Design review of the part built by this model. Coordinates are the model's own, in mm. A direction names the side the tool comes from. Give positions to 0.01 mm unless a question says otherwise; leave off trailing zeros. Order: outer loops, then holes, each group sorted by start corner. A loop starts at its lowest first (then second) coordinate and runs counter-clockwise, first axis right, second up.
```python
from build123d import *

# Parameters (mm, degrees)
BASE_FLANGE1_DEPTH = 40
SKETCH2_R          = 13
CUT_EXTRUDE1_DEPTH = 115.512008104
SKETCH3_R          = 13
CUT_EXTRUDE2_DEPTH = 117.704755687
SKETCH4_R          = 3
CUT_EXTRUDE3_DEPTH = 10
SKETCH5_R          = 3
CUT_EXTRUDE4_DEPTH = 10


# Sheet-metal steps are written as plain solids
with BuildPart() as part:
    # Sketch1 → Base-Flange1 (new body)
    with BuildSketch(Plane.XY):
        with BuildLine():
            Line((0, 0), (-80, 0))
            ThreePointArc((-80, 0), (-82.121320344, -0.878679656), (-83, -3))
            Line((-83, -3), (-83, -68))
            Line((-83, -68), (-86, -68))
            Line((-86, -68), (-86, -3))
            ThreePointArc((-86, -3), (-84.242640687, 1.242640687), (-80, 3))
            Line((-80, 3), (0, 3))
            Line((0, 3), (0, 0))
        make_face()
    extrude(amount=BASE_FLANGE1_DEPTH)

    # Sketch2 → Cut-Extrude1 (cut, through all)
    with BuildSketch(Plane(origin=(-83, 0, 0), x_dir=(0, 0, -1), z_dir=(1, 0, 0))):
        with Locations(Location((-20, -25, 0), (0, 0, 90))):
            Circle(SKETCH2_R)
    extrude(amount=-CUT_EXTRUDE1_DEPTH, mode=Mode.SUBTRACT)

    # Sketch3 → Cut-Extrude2 (cut, through all)
    with BuildSketch(Plane.XZ):
        with Locations((-36, 20)):
            Circle(SKETCH3_R)
    extrude(amount=-CUT_EXTRUDE2_DEPTH, mode=Mode.SUBTRACT)

    # Sketch4 → Cut-Extrude3 (cut)
    with BuildSketch(Plane(origin=(0, 0, 0), x_dir=(-1, 0, 0), z_dir=(0, -1, 0))):
        with Locations(Location((16, -32, 0), (0, 0, 180))):
            Circle(SKETCH4_R)
        with Locations(Location((16, -8, 0), (0, 0, 180))):
            Circle(SKETCH4_R)
    extrude(amount=-CUT_EXTRUDE3_DEPTH, mode=Mode.SUBTRACT)

    # Sketch5 → Cut-Extrude4 (cut)
    with BuildSketch(Plane(origin=(-83, 0, 0), x_dir=(0, 0, -1), z_dir=(1, 0, 0))):
        with Locations(Location((-32, -55, 0), (0, 0, 90))):
            Circle(SKETCH5_R)
        with Locations(Location((-8, -55, 0), (0, 0, 90))):
            Circle(SKETCH5_R)
    extrude(amount=-CUT_EXTRUDE4_DEPTH, mode=Mode.SUBTRACT)


solid = part.part
```
1. Take a section at B-B (x = -16). State the section outline as (y, z) points, then the cut area to 3 significant figures.
Recorded:
outline: (0, 0) - (3, 0) - (3, 5) - (0, 5) - close; (0, 11) - (3, 11) - (3, 29) - (0, 29) - close; (0, 35) - (3, 35) - (3, 40) - (0, 40) - close
area: 84.0 mm2
2. Draft analysis for pull direction Z (two halves, no side actions). For faces 1 (the face through (-84.5, -12.6, 23.9)), 2 (the face through (-62, 2, 40)), 3 (the face through (-83, -42, 20)), state which applies: pulls with the +Z half, pulls with the -Z half, needs draft (parallel to the pull), parting line crosses it, or undercut.
Recorded:
face 1: undercut
face 2: pulls with the +Z half
face 3: needs draft
3. Machinability: for faces 4 (the face through (-84, -58, 32)), 5 (the face through (-48.3, 0, 15.3)), which of the approach directions +Z, -Z, +X, -X, +Y, -Y give a long, thin tool a straight path to every point of the face, cutting with its end or side? Answer none if there is none.
Recorded:
face 4: +X, -X
face 5: +Z, -Z, +X, -Y
4. Take a section at C-C (y = -25). State the section outline as (x, z) points, then the cut area to 3 significant figures.
Recorded:
outline: (-86, 0) - (-83, 0) - (-83, 7) - (-86, 7) - close; (-86, 33) - (-83, 33) - (-83, 40) - (-86, 40) - close
area: 42.0 mm2
5. For pin 1 (9.5 mm diameter, centred on y = -55, z = 8, fed in from +X); pin 2 (3 mm diameter, centred on x = -8.5, z = 31.5, fed in from -Y), all flat-tipped, find the tip position at first contact; note any pin that passes through.
Recorded:
pin 1: stops at x = -83
pin 2: stops at y = 0
6. For line 1 along Z through (x, y) = (-83.55, -55); line 2 along Z through (x, y) = (-85, -25); line 3 along X through (y, z) = (-30, 33), list the stretches that pass through material, from the lowest coordinate up.
Recorded:
line 1: z = 0 to 5, 11 to 29, 35 to 40
line 2: z = 0 to 7, 33 to 40
line 3: x = -86 to -83
7. Take a section at D-D (z = 20). State the section outline as (x, y) points, then the cut area to 3 significant figures.
Recorded:
outline: (-86, -68) - (-83, -68) - (-83, -38) - (-86, -38) - close; (-86, -12) - (-83, -12) - (-83, -3) arc R3 cw to (-80, 0) - (-49, 0) - (-49, 3) - (-80, 3) arc R6 ccw to (-86, -3) - close; (-23, 0) - (0, 0) - (0, 3) - (-23, 3) - close
area: 300 mm2
8. Take a section at A-A (z = 8). State the section outline as (x, y) points, then the cut area to 3 significant figures.
Recorded:
outline: (-86, -68) - (-83, -68) - (-83, -58) - (-86, -58) - close; (-86, -52) - (-83, -52) - (-83, -30) - (-86, -30) - close; (-86, -20) - (-83, -20) - (-83, -3) arc R3 cw to (-80, 0) - (-41, 0) - (-41, 3) - (-80, 3) arc R6 ccw to (-86, -3) - close; (-31, 0) - (-19, 0) - (-19, 3) - (-31, 3) - close; (-13, 0) - (0, 0) - (0, 3) - (-13, 3) - close
area: 360 mm2
